```python
from build123d import *

# Parameters (mm, degrees)
SKETCH_W        = 6
SKETCH_H        = 30
PAD_DEPTH       = 3
SKETCH001_R     = 1.65
POCKET_DEPTH    = 2.5
CHAMFER_SIZE    = 0.4
SKETCH002_W     = 9.60586
SKETCH002_H     = 16.689732
POCKET001_DEPTH = 0.2
CHAMFER001_SIZE = 2


with BuildPart() as part:
    # Sketch → Pad (new body)
    with BuildSketch(Plane.XY):
        Rectangle(SKETCH_W, SKETCH_H)
    extrude(amount=PAD_DEPTH)

    # Sketch001 (on Face6 of Pad) → Pocket (cut)
    with BuildSketch(Plane.XY.offset(3)):
        with Locations((0, 12.2)):
            Circle(SKETCH001_R)
        with Locations((0, -12.2)):
            Circle(SKETCH001_R)
    extrude(amount=-POCKET_DEPTH, mode=Mode.SUBTRACT)

    # Chamfer
    chamfer_edges = [part.edges().sort_by_distance(p)[0] for p in [
        (-1.65, 12.2, 3),
        (-1.65, -12.2, 3),
    ]]
    chamfer(chamfer_edges, length=CHAMFER_SIZE)

    # Sketch002 (on Face1 of Chamfer) → Pocket001 (cut)
    with BuildSketch(Plane.XY.offset(3)):
        Rectangle(SKETCH002_W, SKETCH002_H)
    extrude(amount=-POCKET001_DEPTH, mode=Mode.SUBTRACT)

    # Chamfer001
    chamfer001_edges = [part.edges().sort_by_distance(p)[0] for p in [
        (3, 0, 0),
    ]]
    chamfer(chamfer001_edges, length=CHAMFER001_SIZE)


solid = part.part
```
For this review, take the finished solid that the model builds, in its own axes (mm). A direction names the side the tool comes from. Round coordinates to 2 decimals unless told otherwise and drop trailing zeros. Write each loop counter-clockwise with the first axis right and the second up, starting at its lowest first coordinate (ties: lowest second). Pieces come first, ordered by that corner, then holes. Notation, with made-up numbers: M 15.25,4 L 19.25,4 A29 cw 19.25,28 Z; hole C -16,1.25 d11. An arc over 180 degrees is marked long. One line per item, written item: value. Start each with the question number.
(1) We need section D-D (x = 0). Give the boundary of the cut face in (y, z).
(2) Insertion check: pin 1 (1 mm diameter, centred on x = 2, y = -5.5, fed in from +Z); pin 2 (1.6 mm diameter, centred on x = 0.5, y = -12.5, fed in from +Z). Each pin has a flat end and moves straight along its axis. Give the tip position at first contact, or say it passes through.
(3) Machinability: for faces 4 (the flat face through (0, 0, 2.8)), 5 (the flat face through (0, -15, 1)), which of the approach directions +Z, -Z, +X, -X, +Y, -Y give a long, thin tool a straight path to every point of the face, cutting with its end or side? Answer none if there is none.
(4) The part is to be moulded in two halves that separate along X. For faces 1 (the flat face through (3, -0.2, 2.5)), 2 (the flat face through (-1, -10, 3)), 3 (the flat face through (0, -12, 0.5)), say which applies: released by +X, released by -X, zero draft, split by the parting line, or undercut.
(5) We need section A-A (z = 1.7). Give the boundary of the cut face in (x, y).
(6) We need section B-B (y = -1.75). Give the boundary of the cut face in (x, z).
(7) Wall thickness on line 1 (Y direction, x = 0, z = 1.75); line 2 (Y direction, x = -1.35, z = 2.9); line 3 (Z direction, x = -0.05, y = -2.5): over which ranges is each line inside the solid? List them lowest first.
(8) We need section C-C (x = 2.55). Give the boundary of the cut face in (y, z).
Result:
1. outline: M -15,0 L 15,0 L 15,3 L 14.25,3 L 13.85,2.6 L 13.85,0.5 L 10.55,0.5 L 10.55,2.6 L 10.15,3 L 8.34,3 L 8.34,2.8 L -8.34,2.8 L -8.34,3 L -10.15,3 L -10.55,2.6 L -10.55,0.5 L -13.85,0.5 L -13.85,2.6 L -14.25,3 L -15,3 Z
2. pin 1: z = 2.8
2. pin 2: z = 0.5
3. face 4: +Z, +X, -X
3. face 5: +Z, -Z, +X, -X, -Y
4. face 1: released by +X
4. face 2: zero draft
4. face 3: undercut
5. outline: M -3,-15 L 2.7,-15 L 2.7,15 L -3,15 Z; hole C 0,-12.2 d3.3; hole C 0,12.2 d3.3
6. outline: M -3,0 L 1,0 L 3,2 L 3,2.8 L -3,2.8 Z
7. line 1: -15 to -13.85, -10.55 to 10.55, 13.85 to 15
7. line 2: -15 to -13.61, -10.79 to -8.34, 8.34 to 10.79, 13.61 to 15
7. line 3: 0 to 2.8
8. outline: M -15,1.55 L 15,1.55 L 15,3 L 8.34,3 L 8.34,2.8 L -8.34,2.8 L -8.34,3 L -15,3 Z
